```python
from build123d import *

# Parameters (mm, degrees)
SKETCH1_W               = 42
SKETCH1_H               = 98
BOSS_EXTRUDE1_DEPTH     = 20
SKETCH2_W               = 42
SKETCH2_H               = 70
CUT_EXTRUDE1_DEPTH      = 6
SKETCH3_W               = 42
SKETCH3_H               = 14
BOSS_EXTRUDE2_DEPTH     = 42
FILLET1_R               = 21
CUT_EXTRUDE2_DEPTH      = 74.082145562
CUT_EXTRUDE2_DEPTH_BACK = 74.082145562
SKETCH4_R               = 10
SKETCH6_R               = 6
CUT_EXTRUDE3_DEPTH      = 42
FILLET2_R               = 5


with BuildPart() as part:
    # Sketch1 → Boss-Extrude1 (new body)
    with BuildSketch(Plane(origin=(0, 0, 0), x_dir=(1, 0, 0), z_dir=(0, 1, 0))):
        Rectangle(SKETCH1_W, SKETCH1_H)
    extrude(amount=BOSS_EXTRUDE1_DEPTH)

    # Sketch2 → Cut-Extrude1 (cut)
    with BuildSketch(Plane(origin=(0, 20, 0), x_dir=(1, 0, 0), z_dir=(0, 1, 0))):
        Rectangle(SKETCH2_W, SKETCH2_H)
    extrude(amount=-CUT_EXTRUDE1_DEPTH, mode=Mode.SUBTRACT)

    # Sketch3 → Boss-Extrude2 (add)
    with BuildSketch(Plane.XZ):
        Rectangle(SKETCH3_W, SKETCH3_H)
    extrude(amount=BOSS_EXTRUDE2_DEPTH)

    # Fillet1
    fillet1_edges = [part.edges().sort_by_distance(p)[0] for p in [
        (21, -42, 0),
        (-21, -42, 0),
    ]]
    fillet(fillet1_edges, radius=FILLET1_R - 0.0001)  # a hair under: the kernel refuses the full size

    # Sketch4 → Cut-Extrude2 (cut, two sides: drawn at the far end of the back side and taken through both)
    with BuildSketch(Plane(origin=(0, 0, -7), x_dir=(-1, 0, 0), z_dir=(0, 0, -1)).offset(-CUT_EXTRUDE2_DEPTH_BACK)):
        with Locations((0, -21)):
            Circle(SKETCH4_R)
    extrude(amount=CUT_EXTRUDE2_DEPTH + CUT_EXTRUDE2_DEPTH_BACK, mode=Mode.SUBTRACT)

    # Sketch6 → Cut-Extrude3 (cut)
    with BuildSketch(Plane(origin=(0, 0, 0), x_dir=(1, 0, 0), z_dir=(0, 1, 0))):
        with Locations(Location((0, 25, 0), (0, 0, 90))):
            Circle(SKETCH6_R)
    cut_extrude3 = extrude(amount=CUT_EXTRUDE3_DEPTH, mode=Mode.SUBTRACT)

    # Mirror1: Cut-Extrude3 across plane
    add(cut_extrude3.mirror(Plane.XY), mode=Mode.SUBTRACT)

    # Fillet2
    fillet2_edges = [part.edges().sort_by_distance(p)[0] for p in [
        (0, 0, -7),
        (0, 0, 7),
        (0, 0, -49),
        (0, 0, 49),
    ]]
    fillet(fillet2_edges, radius=FILLET2_R)


solid = part.part
```
Verification items for the finished model (mm, model axes). A direction names the side the tool comes from. Coordinates: 2 decimals unless noted, no trailing zeros. Loops run counter-clockwise (first coordinate to the right, second up) from the corner with the lowest first, then second, coordinate; pieces in that order, holes last. Notation, with made-up numbers: (-2.5, 80) - (21.5, 80) arc R35 ccw to (21.5, 119) - close; hole circle Ø4 at (-11.75, 9.5). An arc over 180 degrees is marked (long way). Return JSON: item names as keys, results as strings.
1. Mould release check, pull along X, two halves, no side actions. Record for faces 1 (the flat face through (-0.3, -31.5, -7)), 2 (the flat face through (-21, 8, 1)), 3 (the cylindrical face through (0, 7, 19)), 4 (the cylindrical face through (0, 7, -19)): +X half, -X half, draft (parallel to the pull), parting line (faces both ways), or undercut.
Established:
{"face 1": "draft", "face 2": "-X half", "face 3": "undercut", "face 4": "undercut"}
2. Section check C-C, the plane x = -8. Record the boundary of the cut face in (y, z), then the cut area to 3 significant figures.
Established:
{"outline": "(-40.42, -7) - (-27, -7) - (-27, 7) - (-40.42, 7) - close; (-15, -7) - (-5, -7) arc R5 cw to (0, -12) - (0, -44) arc R5 ccw to (5, -49) - (20, -49) - (20, -35) - (14, -35) - (14, 35) - (20, 35) - (20, 49) - (5, 49) arc R5 ccw to (0, 44) - (0, 12) arc R5 cw to (-5, 7) - (-15, 7) - close", "area": "1,940 mm2"}
3. Section check A-A, the plane y = 15. Record the boundary of the cut face in (x, z), then the cut area to 3 significant figures.
Established:
{"outline": "(-21, -49) - (21, -49) - (21, -35) - (-21, -35) - close; (-21, 35) - (21, 35) - (21, 49) - (-21, 49) - close", "area": "1,180 mm2"}
4. Go/stop test with flat-tipped pins: pin 1 (12 mm diameter, centred on x = 10, y = -9, fed in from +Z); pin 2 (8 mm diameter, centred on y = -4.5, z = -25, fed in from -X); pin 3 (3 mm diameter, centred on x = 15, z = -4.5, fed in from +Y); pin 4 (23 mm diameter, centred on x = 0, y = -21, fed in from -Z). Record where each tip stops, or that it passes through.
Established:
{"pin 1": "stops at z = 7.42", "pin 2": "passes through", "pin 3": "stops at y = 14", "pin 4": "stops at z = -7"}
5. Tool access check on faces 5 (the flat face through (0, 0, -32)), 6 (the flat face through (-0.3, 0, 31.3)), 7 (the flat face through (0, 12, 49)), 8 (the flat face through (0, 17, -35)). Record the directions out of +Z, -Z, +X, -X, +Y, -Y that give a thin tool (end or side, any length) a straight path to the whole face; none if there is none.
Established:
{"face 5": "-Z, +X, -X, -Y", "face 6": "+Z, +X, -X, -Y", "face 7": "+Z, +X, -X, +Y, -Y", "face 8": "+X, -X, +Y"}
6. Section check D-D, the plane x = 1.5. Record the boundary of the cut face in (y, z), then the cut area to 3 significant figures.
Established:
{"outline": "(-41.95, -7) - (-30.89, -7) - (-30.89, 7) - (-41.95, 7) - close; (-11.11, -7) - (-5, -7) arc R5 cw to (0, -12) - (0, -19.19) - (14, -19.19) - (14, 19.19) - (0, 19.19) - (0, 12) arc R5 cw to (-5, 7) - (-11.11, 7) - close; (0, -44) arc R5 ccw to (5, -49) - (20, -49) - (20, -35) - (14, -35) - (14, -30.81) - (0, -30.81) - close; (0, 30.81) - (14, 30.81) - (14, 35) - (20, 35) - (20, 49) - (5, 49) arc R5 ccw to (0, 44) - close", "area": "1,530 mm2"}
7. Thickness scan on L1, parallel to X at y = 6.5, z = -25; L2, parallel to X at y = -21, z = -2; L3, parallel to Z at x = 10, y = -30. Record the ranges inside material, lowest first.
Established:
{"L1": "x = -21 to -6, 6 to 21", "L2": "x = -21 to -10, 10 to 21", "L3": "z = -7 to 7"}
8. Section check B-B, the plane z = -25. Record the boundary of the cut face in (x, y).
Established:
{"outline": "(-21, 0) - (-6, 0) - (-6, 14) - (-21, 14) - close; (6, 0) - (21, 0) - (21, 14) - (6, 14) - close"}
